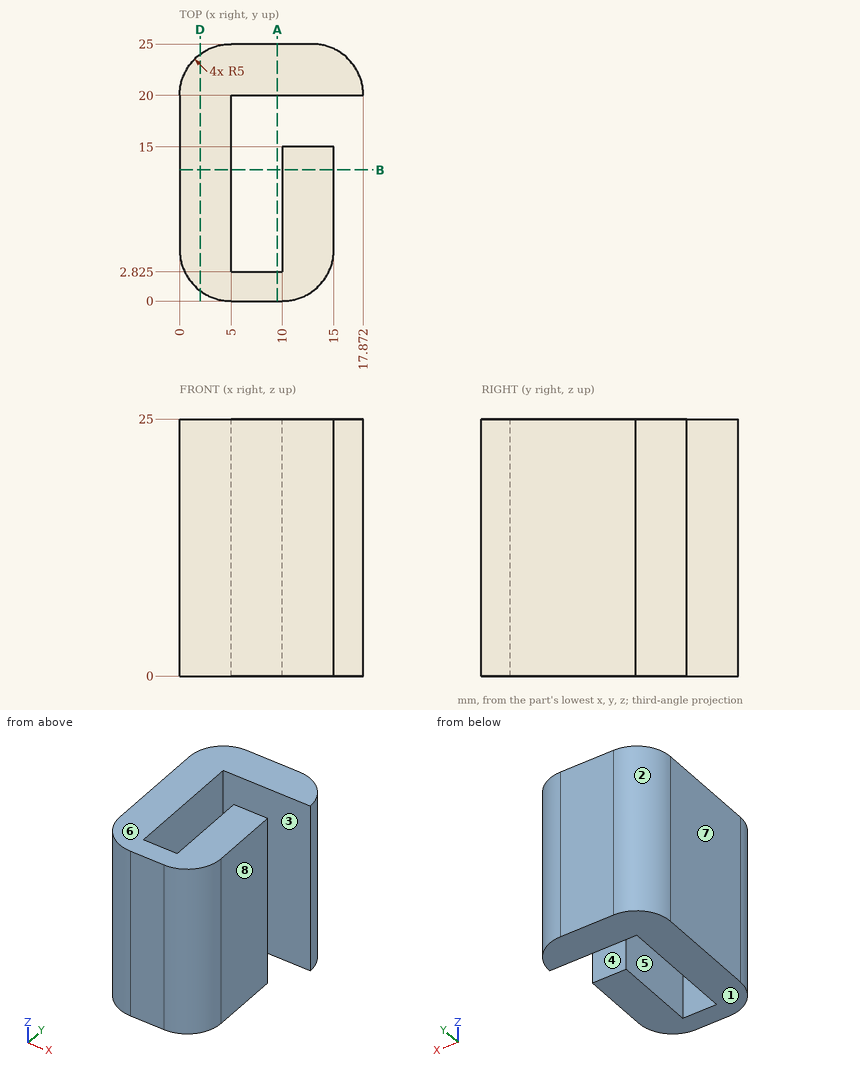
The figure shows three views and two pictorial views of one solid part (mm, origin at its lowest corner). Answer the questions. A direction names the side the tool comes from. Round coordinates to 2 decimals unless told otherwise and drop trailing zeros. Order: outer loops, then holes, each group sorted by start corner. A loop starts at its lowest first (then second) coordinate and runs counter-clockwise, first axis right, second up. Notation, with made-up numbers: M -28,48 L 10,48 A14 ccw 10,72 Z; hole C 41.5,72 d9. An arc over 180 degrees is marked long. Put each result on its own line as item: value. Start each with the question number.
Q1. Section B-B, the plane y = 12.75 is taken. Write down the section's boundary in (x, z).
Q2. Section D-D, the plane x = 2 is taken. Write down the section's boundary in (y, z), and give its area (3 significant figures).
Q3. Straight lines are drawn through the part: L1, parallel to Y at x = 9, z = 5.5 (1 decimal); L2, parallel to X at y = 5.25, z = 11.25; L3, parallel to Y at x = 12.25, z = 9.5 (1 decimal). For each, find the intervals that lie inside material, in ascending order. Write a range as [from, to].
Q4. Flat-ended cylindrical pins translate along their axes: pin 1 (8 mm diameter, centred on y = 19, z = 18.5, fed in from -X); pin 2 (1 mm diameter, centred on x = 3.5, z = 18, fed in from -Y); pin 3 (1 mm diameter, centred on y = 6.5, z = 14.5, fed in from +X). Find the tip coordinate at first contact, or state that the pin passes through.
Q5. A tool of negligible diameter and unlimited length cuts with its end or side. For the marked faces 4, 5, 6, 7 and 8, from which of +Z, -Z, +X, -X, +Y, -Y can it reach the whole face along a straight path? Write none if from no direction.
Q6. For a pull along Y with two mould halves and no side action, classify the marked faces 1, 2 and 3 as pulls with the +Y half, pulls with the -Y half, needs draft (parallel to the pull), parting line crosses it, or undercut.
Q7. Section A-A, the plane x = 9.5 is taken. Write down the section's boundary in (y, z) (1 decimal), and give its area (3 significant figures).
Findings below:
1. outline: M 0,0 L 5,0 L 5,25 L 0,25 Z; M 10,0 L 15,0 L 15,25 L 10,25 Z
2. outline: M 1,0 L 24,0 L 24,25 L 1,25 Z
2. area: 575 mm^2
3. L1: y = [0, 2.8], [20, 25]
3. L2: x = [0, 5], [10, 15]
3. L3: y = [0.5, 15], [20, 25]
4. pin 1: stops at x = 0
4. pin 2: stops at y = 0.1
4. pin 3: stops at x = 15
5. face 4: +Z, -Z, +X
5. face 5: +Z, -Z
5. face 6: +Z, +X, -X, +Y, -Y
5. face 7: +Z, -Z, -X, +Y, -Y
5. face 8: +Z, -Z, +X, -Y
6. face 1: needs draft
6. face 2: pulls with the +Y half
6. face 3: undercut
7. outline: M 0,0 L 2.8,0 L 2.8,25 L 0,25 Z; M 20,0 L 25,0 L 25,25 L 20,25 Z
7. area: 196 mm^2
